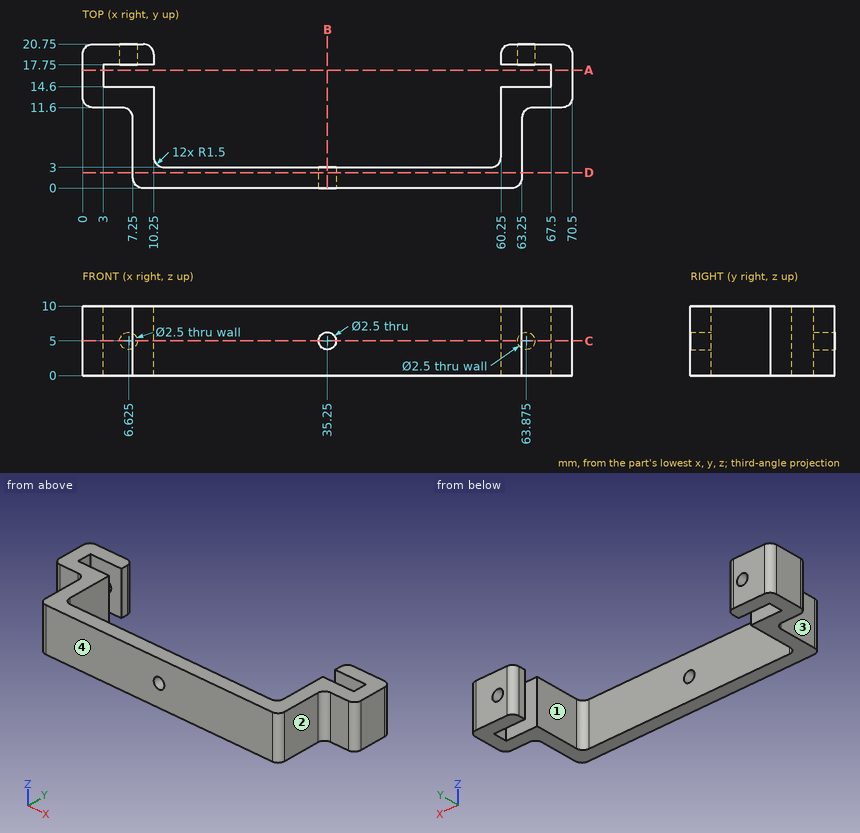
Can you work these out from the drawing? Everything is in mm from the part's minimum corner. A direction names the side the tool comes from. Round coordinates to 2 decimals unless told otherwise and drop trailing zeros. Order: outer loops, then holes, each group sorted by start corner. A loop starts at its lowest first (then second) coordinate and runs counter-clockwise, first axis right, second up. Notation, with made-up numbers: (9.25, 62) - (54.25, 62) arc R13 cw to (54.25, 73) - close; hole circle Ø10 at (61, 71). An arc over 180 degrees is marked (long way). Answer in a Markdown table with one row per item.
(1) For P1, Ø6, axis at x = 62, z = 4.5, coming from the -Y side; P2, Ø2, axis at x = 4, z = 3, coming from the -Y side; P3, Ø5, axis at y = 9.5, z = 7, coming from the -X side; P4, Ø1.5, axis at x = 35.25, z = 5, coming from the +Y side, each with a flat end and sliding along its axis, tell me the tip position at first contact or that it passes through.
From the geometry:
| item | result |
|---|---|
| P1 | stops at y = 0 |
| P2 | stops at y = 11.6 |
| P3 | stops at x = 0.48 |
| P4 | passes through |
(2) Suppose I cut it at B-B, the plane x = 35.25. Please give me the cut outline in (y, z).
From the geometry:
| item | result |
|---|---|
| outline | (0, 0) - (3, 0) - (3, 3.75) - (0, 3.75) - close; (0, 6.25) - (3, 6.25) - (3, 10) - (0, 10) - close |
(3) Please list where these lines run through material, in increasing order: L1, parallel to X at y = 18.8, z = 5 (3 decimals); L2, parallel to X at y = 7.75, z = 2.75; L3, parallel to X at y = 19.9, z = 5 (3 decimals). Write a range as from..to.
From the geometry:
| item | result |
|---|---|
| L1 | x = 0..5.375, 7.875..10.25, 60.25..62.625, 65.125..70.5 |
| L2 | x = 7.25..10.25, 60.25..63.25 |
| L3 | x = 0.148..5.375, 7.875..10.102, 60.398..62.625, 65.125..70.352 |
(4) Which directions (+Z, -Z, +X, -X, +Y, -Y) give clear straight access to the entire face, cutting with the end or side of a thin tool? Please do the marked faces 1, 2, 3 and 4.
From the geometry:
| item | result |
|---|---|
| face 1 | +Z, -Z, +Y |
| face 2 | +Z, -Z, +X, -Y |
| face 3 | +Z, -Z, -X, -Y |
| face 4 | +Z, -Z, +X, -X, -Y |
(5) Suppose I cut it at A-A, the plane y = 17. Please give me the cut outline in (x, z).
From the geometry:
| item | result |
|---|---|
| outline | (0, 0) - (3, 0) - (3, 10) - (0, 10) - close; (67.5, 0) - (70.5, 0) - (70.5, 10) - (67.5, 10) - close |
(6) Suppose I cut it at D-D, the plane y = 2.25. Please give me the cut outline in (x, z), plus the area to 3 significant figures.
From the geometry:
| item | result |
|---|---|
| outline | (7.25, 0) - (63.25, 0) - (63.25, 10) - (7.25, 10) - close; hole circle Ø2.5 at (35.25, 5) |
| area | 555 mm2 |
(7) Suppose I cut it at C-C, the plane z = 5. Count the separate pieces of the cut face and the enclosed holes in it, plus the area to 3 significant figures.
From the geometry:
| item | result |
|---|---|
| separate pieces | 4 |
| enclosed holes | 0 |
| area | 337 mm2 |
